Autodesk Inventor part; units mm, degrees
ref_plane "YZ Plane" through (0, 0, 0) normal (1, 0, 0) x (0, 1, 0)
ref_plane "XZ Plane" through (0, 0, 0) normal (0, 1, 0) x (-1, 0, 0)
ref_plane "XY Plane" through (0, 0, 0) normal (0, 0, 1) x (1, 0, 0)
sketch "Sketch1" plane through (0, 0, 0) normal (0, 1, 0) x (-1, 0, 0)
  circle A0 centre (0, 0) radius 213
  circle A1 centre (0, 0) radius 270
  line L0 (270, 0) -> (213, 0)
  line L1 (-213, 0) -> (-270, 0)
  line L2 (0, 213) -> (0, 270)
  point P0 (241.5, 0)
  point P1 (-241.5, 0)
  point P2 (0, 241.5)
  dimension "d1" = 540
  dimension "d4" = 426
extrude "Extrusion1" add sketch "Sketch1" along normal blind 6 contours L0 A1 L1 A0 | A0 L2 A1 L0 | A0 L1 A1 L2
sketch "Sketch2" plane through (0, 0, 0) normal (0, -1, 0) x (1, 0, 0)
  circle A0 centre (0, 0) radius 270
  circle A1 centre (0, 0) radius 213
  circle A2 centre (38.7175, 244.4529) radius 11
  circle A3 centre (0, 0) radius 213
  line L0 (38.7175, 244.4529) -> (0, 0)
  point P0 (0, 213)
  point P1 (265, 0)
  dimension "d5" = 247.5
  dimension "d7" = 22
extrude "Cut1" cut sketch "Sketch2" against normal blind 6 contours A2
pattern_circular "Circular Pattern1" count 16 over 360 about axis through (0, 0, 0) along (0, 1, 0) of "Cut1"
equation "\"d1\" = Charging_hatch_width"
equation "\"d4\" = Accsess_hatch_diameter"
equation "\"d9\" = Thickness"
equation "\"BendRadius\" = Thickness"
equation "\"BendReliefWidth\" = Thickness"
equation "\"BendReliefDepth\" = 0.5 * Thickness"
equation "\"CornerReliefSize\" = 4 * Thickness"
equation "\"MinimumRemnant\" = 2 * Thickness"
equation "\"TransitionRadius\" = BendRadius"
equation "\"JacobiRadiusSize\" = BendRadius"
equation "\"GapSize\" = Thickness"
equation "\"d8\" = Thickness"
properties part number "TZS 0903 accses hatch flange" material "Steel"
CAD build for the part. Positions are in the model's coordinates, mm. Round coordinates to 2 decimals unless told otherwise and drop trailing zeros. Write each loop counter-clockwise with the first axis right and the second up, starting at its lowest first coordinate (ties: lowest second). Pieces come first, ordered by that corner, then holes.
(1) Probe line 1 along X through (y, z) = (4.1, 129); line 2 along Z through (x, y) = (-60.5, 0.5); line 3 along X through (y, z) = (4.45, -65.5). List the from-to ranges inside material, lowest first.
(2) Mould opens along Z. For faces 1 (the face through (214.263, 2.958, 164.291)), 2 (the face through (-79, 6, 201)), 3 (the face through (233.714, 2.958, -36.333)) say: pulls with the +Z half, pulls with the -Z half, needs draft (parallel to the pull), parting line crosses it, or undercut.
(3) Slice it at A-A, the plane x = 0. Write the cut outline in (y, z), and give its area (3 significant figures).
(4) Slice it at B-B, the plane z = 0. Write the cut outline in (x, y), and give its area (3 significant figures).
(5) Slice it at C-C, the plane x = 148.5. Write the cut outline in (y, z).
(6) Drop flat-ended pins along their axis: P1, Ø1.5, axis at x = -42.5, y = 4.5, coming from the +Z side; P2, Ø13, axis at x = -244.45, z = 38.72, coming from the +Y side. Give the stop position or say it passes through.
From the geometry:
1. line 1: x = -237.19 to -222.02, -200.03 to -169.49, 169.49 to 237.19
1. line 2: z = -263.13 to -204.23, 204.23 to 230, 251.32 to 263.13
1. line 3: x = -261.93 to -248.5, -232.83 to -202.68, 202.68 to 261.93
2. face 1: parting line crosses it
2. face 2: needs draft
2. face 3: undercut
3. outline: (0, -270) - (6, -270) - (6, -213) - (0, -213) - close; (0, 213) - (6, 213) - (6, 270) - (0, 270) - close
3. area: 684 mm2
4. outline: (-270, 0) - (-213, 0) - (-213, 6) - (-270, 6) - close; (213, 0) - (270, 0) - (270, 6) - (213, 6) - close
4. area: 684 mm2
5. outline: (0, -225.49) - (6, -225.49) - (6, -210.81) - (0, -210.81) - close; (0, -189.66) - (6, -189.66) - (6, -152.7) - (0, -152.7) - close; (0, 152.7) - (6, 152.7) - (6, 225.49) - (0, 225.49) - close
6. P1: stops at z = 266.75
6. P2: passes through
